The listing builds one solid part. Answer for the finished solid, in the listing's coordinates (mm). Face numbers are marked on the shaded views. A direction names the side the tool comes from. Give positions to 0.01 mm unless a question says otherwise; leave off trailing zeros. Order: outer loops, then holes, each group sorted by start corner. A loop starts at its lowest first (then second) coordinate and runs counter-clockwise, first axis right, second up. Notation, with made-up numbers: (76.25, -19.75) -> (125.25, -19.75) arc R25 ccw to (125.25, -4.75) -> close; hole circle Ø8 at (18.25, 27). An arc over 180 degrees is marked (long way). Write item = value, one per line. Start each with the question number.
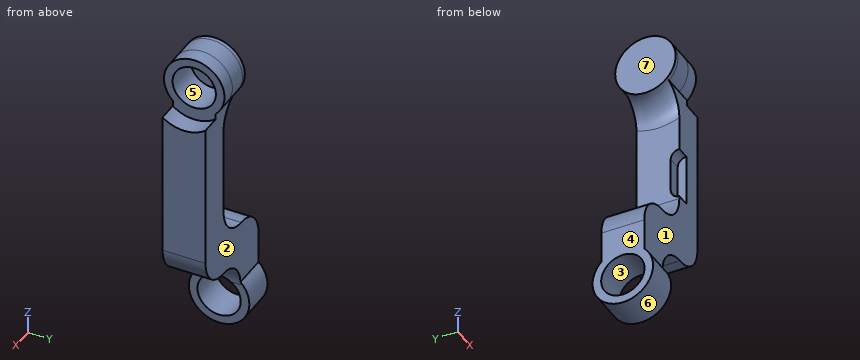
Autodesk Inventor part; units mm, degrees
ref_plane "YZ Plane" through (0, 0, 0) normal (1, 0, 0) x (0, 1, 0)
ref_plane "XZ Plane" through (0, 0, 0) normal (0, 1, 0) x (-1, 0, 0)
ref_plane "XY Plane" through (0, 0, 0) normal (0, 0, 1) x (1, 0, 0)
sketch "Эскиз1" plane through (0, 0, 0) normal (0, 1, 0) x (-1, 0, 0)
  line L0 (0, 0) -> (4, 0)
  line L1 (4, 0) -> (4, -23.9397)
  line L2 (4, -23.9397) -> (0, -23.9397)
  line L3 (0, -23.9397) -> (0, 0)
  line L4 (0, -23.9397) -> (11.75, -23.9397)
  line L5 (11.75, -23.9397) -> (11.75, -19.9397)
  line L6 (11.75, -19.9397) -> (0, -19.9397)
  line L7 (0, -19.9397) -> (0, -23.9397)
  line L8 (11.75, -19.9397) -> (7.75, -19.9397)
  line L9 (7.75, -19.9397) -> (7.75, -29.9397)
  line L10 (7.75, -29.9397) -> (11.75, -29.9397)
  line L11 (11.75, -29.9397) -> (11.75, -19.9397)
  line L12 (11.75, -23.9397) -> (4, -19.9397)
  line L13 (0, -19.9397) -> (7.75, -23.9397)
  point P0 (3, -20.536)
  point P1 (0, -19.9397)
  dimension "d10" = 4
  dimension "d11" = 11.75
  dimension "d36" = 29.9397
  dimension "d57" = 10
extrude "Выдавливание1" add sketch "Эскиз1" along normal blind 5
fillet "Сопряжение2" radius 3.855 4 edges at (-4, 2.5, -19.9397) (-11.75, 2.5, -19.9397) (0, 2.5, -23.9397) (-7.75, 2.5, -23.9397)
sketch "Эскиз7" plane through (-11.75, 0, -29.9397) normal (-1, 0, 0) x (0, 0, 1)
  line L0 (0, 0) -> (0, 5)
  circle A0 centre (0, 2.5) radius 2.525
  circle A1 centre (0, 2.5) radius 3.525
  point P0 (29.9397, 0)
  point P1 (0, 4.975)
  point P2 (0, 0.025)
  dimension "d37" = 5.05
  dimension "d38" = 7.05
extrude "Выдавливание5" add sketch "Эскиз7" against normal up to surface (4 mm away) contours A0 | A1
extrude "Выдавливание8" cut sketch "Эскиз7" against normal through all contours A0
sketch "Эскиз8" plane through (-4, 0, 0) normal (-1, 0, 0) x (0, 0, 1)
  line L0 (0, 0) -> (0, 5)
  circle A0 centre (0, 2.5) radius 2.525
  circle A1 centre (0, 2.5) radius 3.525
  point P0 (0, 4.975)
  point P1 (0, 0.025)
  dimension "d41" = 5.05
  dimension "d42" = 7.05
extrude "Выдавливание6" add sketch "Эскиз8" against normal up to surface (4 mm away)
extrude "Выдавливание7" cut sketch "Эскиз8" against normal through all contours A0
sketch "Эскиз9" plane through (0, 0, -20.0847) normal (1, 0, 0) x (0, 0, -1)
  arc A0 (-19.7302, 5) -> (-19.7302, 0) centre (-20.0847, 2.5) ccw
  circle A1 centre (-20.0847, 2.5) radius 4.025
  arc A2 (-17.5996, 5) -> (-17.5996, 0) centre (-20.0847, 2.5) ccw
  point P0 (-20.0847, 0)
  point P1 (-20.0847, 4.975)
  point P2 (-20.0847, 0.025)
  dimension "d49" = 0.5
extrude "Выдавливание9" cut sketch "Эскиз9" against normal blind 2.25
sketch "Эскиз10" plane through (-4, 0, -16.0847) normal (-1, 0, 0) x (0, 0, 1)
  arc A0 (13.5996, 0) -> (13.5996, 5) centre (16.0847, 2.5) ccw
  circle A1 centre (16.0847, 2.5) radius 3.525
  circle A2 centre (16.0847, 2.5) radius 2.525
  point P0 (16.0847, 0)
  point P1 (13.5996, 5)
  point P2 (13.5996, 0)
extrude "Выдавливание10" add sketch "Эскиз10" along normal blind 2.25
sketch "Эскиз11" plane through (-6.25, 2.5, 0) normal (-1, 0, 0) x (0, 0, 1)
  circle A0 centre (0, 0) radius 3.525
  point P0 (0, -2.5)
extrude "Выдавливание11" add sketch "Эскиз11" along normal blind 0.5
fillet "Сопряжение6" radius 2.75 1 edges at (-4, 2.5, -3.525)
sketch "Эскиз12" plane through (-4, 0, -16.0847) normal (-1, 0, 0) x (0, 0, 1)
  line L0 (5.3292, 0) -> (1.3292, 0) construction
  line L1 (5.3292, 1) -> (1.3292, 1)
  line L2 (1.3292, -1) -> (5.3292, -1)
  arc A0 (5.3292, -1) -> (5.3292, 1) centre (5.3292, 0) ccw
  arc A1 (1.3292, 1) -> (1.3292, -1) centre (1.3292, 0) ccw
  line L3 (0, 0) -> (10.3292, 0)
  point P0 (16.0847, 0)
  point P1 (3.3292, 0)
  dimension "d58" = 2
  dimension "d59" = 2
  dimension "d63" = 7
extrude "Выдавливание12" cut sketch "Эскиз12" against normal blind 1.55
properties part number "Рулевая тяга"
Item 1: The mould has two halves that part along Y. Classify the marked faces 1, 2, 3 and 4: +Y half, -Y half, draft (parallel to the pull), parting line (faces both ways), or undercut.
Item 2: Consider L1, parallel to Z at x = -3.65, y = 2.5 (3 decimals); L2, parallel to Y at x = -3.75, z = 0 (3 decimals); L3, parallel to Z at x = -5.25, y = 3.25. Determine where each line is inside the solid, lowest interval first. Write a range as from..to.
Item 3: A cutting plane is placed at C-C, the plane z = 0. Write down the section's boundary in (x, y) (3 decimals).
Item 4: A cutting plane is placed at B-B, the plane x = -5.5. Write down the section's boundary in (y, z) (3 decimals).
Item 5: A cutting plane is placed at A-A, the plane y = 2.5. Write down the section's boundary in (x, z) (3 decimals), plus the area to 3 significant figures.
Item 6: A cutting plane is placed at D-D, the plane x = -9.5. Write down the section's boundary in (y, z) (3 decimals).
Item 7: Flat-ended cylindrical pins translate along their axes: pin 1 (1.8 mm diameter, centred on y = 4, z = -31, fed in from +X); pin 2 (2.5 mm diameter, centred on y = 1.5, z = -13, fed in from -X); pin 3 (0.5 mm diameter, centred on y = 0.5, z = -12.5, fed in from -X); pin 4 (3 mm diameter, centred on x = -2.5, y = 1, fed in from +Z) (3 decimals). Find the tip coordinate at first contact, or state that the pin passes through.
Item 8: Which of the six approach directions +Z, -Z, +X, -X, +Y, -Y give full straight-line access (tool end or side, diameter ignored) to the marked faces 5, 6 and 7?
Check values:
q1.face_1 = -Y half
q1.face_2 = +Y half
q1.face_3 = undercut
q1.face_4 = draft
q2.L1 = -23.934..-2.525, 2.525..3.525
q2.L2 = -1.025..-0.025, 5.025..6.025
q2.L3 = -24.19..-18.93, -3.9..-2.41, 2.41..3.44
q3.outline = (-6.75, -1.025) -> (-6.25, -1.025) -> (-2.25, -1.025) -> (-2.25, -0.025) -> (-6.25, -0.025) -> (-6.25, 5.025) -> (-2.25, 5.025) -> (-2.25, 6.025) -> (-6.25, 6.025) -> (-6.75, 6.025) -> close
q4.outline = (0, -24.29) -> (5, -24.29) -> (5, -19.137) -> (0, -19.137) -> close; (0, -2.896) arc R3.826 ccw to (5, -2.896) -> (5, -2.485) arc R3.525 ccw (long way) to (0, -2.485) -> close; hole circle Ø5.05 at (2.5, 0)
q5.outline = (-11.75, -33.465) -> (-7.75, -33.465) -> (-7.75, -32.465) -> (-11.75, -32.465) -> close; (-11.75, -27.415) -> (-7.731, -27.415) arc R3.855 cw to (-3.895, -23.94) -> (-3.855, -23.94) arc R3.855 ccw to (0, -20.085) -> (0, -4.025) -> (-2.25, -4.025) -> (-2.25, -2.525) -> (-6.25, -2.525) -> (-6.25, 2.525) -> (-2.25, 2.525) -> (-2.25, 3.525) -> (-4, 3.525) -> (-6.75, 3.525) -> (-6.75, -3.525) arc R2.75 cw to (-4, -6.275) -> (-4, -16.085) arc R3.855 cw to (-7.855, -19.94) -> (-7.895, -19.94) arc R3.855 ccw to (-11.75, -23.795) -> close
q5.area = 143 mm^2
q6.outline = (0, -27.455) arc R3.525 ccw (long way) to (5, -27.455) -> (5, -20.29) -> (0, -20.29) -> close; hole circle Ø5.05 at (2.5, -29.94)
q7.pin_1 = -7.75
q7.pin_2 = -4
q7.pin_3 = -2.45
q7.pin_4 = 3.525
q8.face_5 = +X
q8.face_6 = +X, -X
q8.face_7 = +Z, -X, +Y, -Y
